Design review of the part built by this model. Coordinates are the model's own, in mm. Face numbers are marked on the shaded views. Round coordinates to 2 decimals unless told otherwise and drop trailing zeros. Loops run counter-clockwise (first coordinate to the right, second up) from the corner with the lowest first, then second, coordinate; pieces in that order, holes last. Notation, with made-up numbers: (55, 56.25) - (107, 56.25) arc R25 cw to (107, 88.25) - close; hole circle Ø2 at (88, -26.75). An arc over 180 degrees is marked (long way). Answer as CSV lines item,"result". Start each with the question number.
(1) Wall thickness on L1, parallel to Y at x = -13, z = 21; L2, parallel to Y at x = 8, z = 10; L3, parallel to Z at x = -0.5, y = 40: over which ranges is each line inside the solid? List them lowest first.
(2) Consider section B-B (x = 21.5). Give the boundary of the cut face in (y, z), and give its area (3 significant figures).
(3) Mouldability with a two-part tool opening along X and no side actions: class the marked faces 1, 2 and 3 as released by +X, released by -X, zero draft, split by the parting line, or undercut.
(4) Consider section A-A (y = 26.5). Count the separate pieces of the cut face and the enclosed holes in it, and give its area (3 significant figures).
(5) For P1, Ø8, axis at y = 19, z = -20.5, coming from the -X side; P2, Ø0.8, axis at y = 29, z = 24, coming from the -X side; P3, Ø5, axis at x = 9, y = 53, coming from the -Z side, all flat-tipped, find the tip position at first contact; note any pin that passes through.
from build123d import *

# Parameters (mm, degrees)
SKETCH_1_R               = 10
EXTRUDE_1_DEPTH          = 3
EXTRUDE_1_TAPER          = 35
SKETCH_2_W               = 4
SKETCH_2_H               = 17
EXTRUDE_2_DEPTH          = 2
PATTERN_CIRCULAR_1_COUNT = 8
SKETCH_3_R               = 25
SKETCH_3_R_2             = 22.5
EXTRUDE_3_DEPTH          = 2
SKETCH_5_W               = 4
SKETCH_5_H               = 1
EXTRUDE_4_DEPTH          = 60
PATTERN_CIRCULAR_2_COUNT = 14
SKETCH_8_R               = 25.353025185
SKETCH_8_R_2             = 24.353025185
EXTRUDE_1_2_DEPTH        = 24
SKETCH_9_R               = 26.182989569
SKETCH_9_R_2             = 25.182989569
EXTRUDE_2_2_DEPTH        = 3


with BuildPart() as part:
    # Эскиз1 → Extrude 1 (new body)
    with BuildSketch(Plane(origin=(0, 0, 0), x_dir=(1, 0, 0), z_dir=(0, 1, 0))):
        Circle(SKETCH_1_R)
    extrude(amount=EXTRUDE_1_DEPTH, taper=EXTRUDE_1_TAPER)

    # Эскиз2 → Extrude 2 (add)
    with BuildSketch(Plane.XZ):
        with Locations((0, 15.5)):
            Rectangle(SKETCH_2_W, SKETCH_2_H)
    extrude_2 = extrude(amount=-EXTRUDE_2_DEPTH)

    # Круговой массив1: Extrude 2 ×8 about axis
    pattern_circular_1_axis = Axis((0, 0, 0), (0, 1, 0))
    for i in range(1, PATTERN_CIRCULAR_1_COUNT):
        add(extrude_2.rotate(pattern_circular_1_axis, i * 360 / PATTERN_CIRCULAR_1_COUNT))

    # Эскиз3 → Бобышка-Вытянуть3 (add)
    with BuildSketch(Plane(origin=(0, 0, 0), x_dir=(1, 0, 0), z_dir=(0, 1, 0))):
        with Locations(Location((0, 0, 0), (0, 0, 270))):
            Circle(SKETCH_3_R)
        Circle(SKETCH_3_R_2, mode=Mode.SUBTRACT)
    extrude(amount=EXTRUDE_3_DEPTH)

    # Эскиз5 → Бобышка-Вытянуть4 (add)
    with BuildSketch(Plane(origin=(0, 2, 0), x_dir=(1, 0, 0), z_dir=(0, 1, 0))):
        with Locations((-0.12233464, 23.853025185)):
            Rectangle(SKETCH_5_W, SKETCH_5_H)
    extrude_4 = extrude(amount=EXTRUDE_4_DEPTH)

    # Круговой массив2: Бобышка-Вытянуть4 ×14 about axis
    pattern_circular_2_axis = Axis((0, 0, 0), (0, 1, 0))
    for i in range(1, PATTERN_CIRCULAR_2_COUNT):
        add(extrude_4.rotate(pattern_circular_2_axis, i * 360 / PATTERN_CIRCULAR_2_COUNT))

    # Эскиз8 → Extrude 1 2 (add)
    with BuildSketch(Plane(origin=(0, 62, 0), x_dir=(1, 0, 0), z_dir=(0, 1, 0))):
        Circle(SKETCH_8_R)
        Circle(SKETCH_8_R_2, mode=Mode.SUBTRACT)
    extrude(amount=-EXTRUDE_1_2_DEPTH)

    # Эскиз9 → Extrude 2 2 (add)
    with BuildSketch(Plane(origin=(0, 62, 0), x_dir=(1, 0, 0), z_dir=(0, 1, 0))):
        Circle(SKETCH_9_R)
        Circle(SKETCH_9_R_2, mode=Mode.SUBTRACT)
    extrude(amount=-EXTRUDE_2_2_DEPTH)


solid = part.part
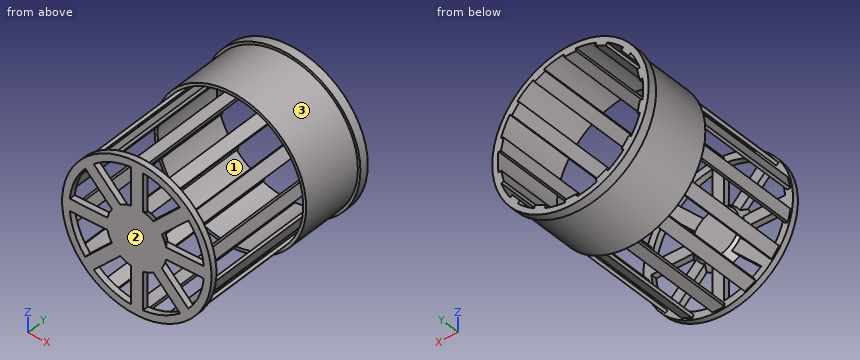
Determined:
1,L1,"y = 0 to 2, 38 to 62"
1,L2,"y = 0 to 2"
1,L3,"z = -25.35 to -23.35, 23.35 to 25.35"
2,outline,"(0, -12.76) - (2, -12.76) - (2, -6.63) - (0, -6.63) - close; (0, -2) - (2, -2) - (2, 2) - (0, 2) - close; (0, 6.63) - (2, 6.63) - (2, 12.76) - (0, 12.76) - close; (38, -13.44) - (59, -13.44) - (59, -14.94) - (62, -14.94) - (62, -11.44) - (38, -11.44) - close; (38, 11.44) - (62, 11.44) - (62, 14.94) - (59, 14.94) - (59, 13.44) - (38, 13.44) - close"
2,area,"137 mm^2"
3,face 1,"undercut"
3,face 2,"zero draft"
3,face 3,"split by the parting line"
4,separate pieces,"14"
4,enclosed holes,"0"
4,area,"56.0 mm^2"
5,P1,"stops at x = -17.99"
5,P2,"stops at x = -1.88"
5,P3,"stops at z = -24.51"
